Check sheet for the modelled part. Datum: model origin and axes. Units: mm. A direction names the side the tool comes from. Round coordinates to 2 decimals unless told otherwise and drop trailing zeros. Write each loop counter-clockwise with the first axis right and the second up, starting at its lowest first coordinate (ties: lowest second). Pieces come first, ordered by that corner, then holes. Notation, with made-up numbers: (2.25, 34.25) -> (60.25, 34.25) arc R19 cw to (60.25, 63.25) -> close; hole circle Ø6 at (10, -3). An arc over 180 degrees is marked (long way). Write item = value, one per line.
from build123d import *

# Parameters (mm, degrees)
CHAMFER1_SIZE      = 0.993775
CHAMFER2_SIZE      = 0.46434375
CHAMFER3_SIZE      = 0.2032
CUT_EXTRUDE2_DEPTH = 3.175


with BuildPart() as part:
    # Sketch1 → Revolve1 (revolve)
    with BuildSketch(Plane(origin=(0, 0, 0), x_dir=(0, 0, -1), z_dir=(1, 0, 0))):
        Polygon((0, 7.14375), (6.35, 7.14375), (6.35, 4.7625), (69.85, 4.7625), (69.85, 3.9751), (82.55, 3.9751), (82.55, 0), (0, 0), align=None)
    revolve(axis=Axis((0, 0, -82.55), (0, 0, 1)))

    # Sketch5 → Cut-Revolve1 (revolve, cut)
    with BuildSketch(Plane(origin=(0, 0, 0), x_dir=(0, 0, -1), z_dir=(1, 0, 0))):
        with BuildLine():
            Line((69.85, 4.7625), (74.422, 4.7625))
            Line((74.422, 4.7625), (72.6694, 3.0099))
            Line((72.6694, 3.0099), (70.8152, 3.0099))
            ThreePointArc((70.8152, 3.0099), (70.132700535, 3.292600535), (69.85, 3.9751))
            Line((69.85, 3.9751), (69.85, 4.7625))
        make_face()
    revolve(axis=Axis((0, 0, -82.55), (0, 0, 1)), mode=Mode.SUBTRACT)

    # Chamfer1
    chamfer1_edges = [part.edges().sort_by_distance(p)[0] for p in [
        (0, -3.9751, -82.55),
    ]]
    chamfer(chamfer1_edges, length=CHAMFER1_SIZE)

    # Chamfer2
    chamfer2_edges = [part.edges().sort_by_distance(p)[0] for p in [
        (0, -7.14375, 0),
    ]]
    chamfer(chamfer2_edges, length=CHAMFER2_SIZE)

    # Chamfer3
    chamfer3_edges = [part.edges().sort_by_distance(p)[0] for p in [
        (0, -4.7625, -69.85),
    ]]
    chamfer(chamfer3_edges, length=CHAMFER3_SIZE)

    # Sketch8 → Cut-Extrude2 (cut)
    with BuildSketch(Plane.XY):
        Polygon((2.38125, 1.374815329), (0, 2.749630657), (-2.38125, 1.374815329), (-2.38125, -1.374815329), (0, -2.749630657), (2.38125, -1.374815329), align=None)
    extrude(amount=-CUT_EXTRUDE2_DEPTH, mode=Mode.SUBTRACT)

    # Cut-Extrude4 cone 1 section (through the dimple's axis) → Cut-Extrude4 (revolve, cut)
    with BuildSketch(Plane(origin=(0, 0, 0), x_dir=(0, -1, 0), z_dir=(1, 0, 0))):
        Polygon((0, 0), (2.749630657, 0), (0, 2.749630657), align=None)
    revolve(axis=Axis((0, 0, 0), (0, 0, -1)), mode=Mode.SUBTRACT)

    # Sketch12 → Revolve2 (revolve)
    with BuildSketch(Plane(origin=(0, 0, 0), x_dir=(0, 0, -1), z_dir=(1, 0, 0))):
        with BuildLine():
            Line((69.85, 4.5593), (69.6468, 4.7625))
            Line((69.6468, 4.7625), (6.35, 4.7625))
            Line((6.35, 4.7625), (6.35, 0))
            Line((6.35, 0), (69.85, 0))
            Line((69.85, 0), (72.6694, 0))
            Line((72.6694, 0), (72.6694, 3.0099))
            Line((72.6694, 3.0099), (70.8152, 3.0099))
            ThreePointArc((70.8152, 3.0099), (70.132700535, 3.292600535), (69.85, 3.9751))
            Line((69.85, 3.9751), (69.85, 4.5593))
        make_face()
    revolve(axis=Axis((0, 0, -6.35), (0, 0, -1)))


solid = part.part
(1) Sectioned sample at B-B on z = -33.5. Enter the section's corners in (x, y) (1 decimal).
Worked answers:
outline = circle Ø9.5 at (0, 0)
(2) Access from +Z, -Z, +X, -X, +Y, -Y to the whole of each face (thin tool, end or side, straight path). Record for faces 1 (the flat face through (0, -3, 0)), 2 (the flat face through (1.174, -2.072, -1.565)), 3 (the cylindrical face through (3.88, -0.86, -77.65)).
Worked answers:
face_1 = +Z, +X, -X, +Y, -Y
face_2 = +Z
face_3 = -Z
(3) Release check for a two-part mould opening along Z. For faces 4 (the cylindrical face through (1.83, -2.39, -71.73)), 5 (the conical face through (-1.298, 2.21, -0.187)), 6 (the cylindrical face through (2.9, -3.78, -38.44)) record: pulls with the +Z half, pulls with the -Z half, needs draft (parallel to the pull), parting line crosses it, or undercut.
Worked answers:
face_4 = undercut
face_5 = pulls with the +Z half
face_6 = needs draft
(4) Go/stop test with flat-tipped pins: P1, Ø8, axis at y = 2, z = -18.5, coming from the +X side; P2, Ø6, axis at x = 2.5, z = -42, coming from the -Y side; P3, Ø6, axis at x = -5, z = -18.5, coming from the +Y side. Record where each tip stops, or that it passes through.
Worked answers:
P1 = 4.76
P2 = -4.76
P3 = 4.32
(5) Sectioned sample at C-C on z = -75. Enter the section's corners in (x, y).
Worked answers:
outline = circle Ø7.95 at (0, 0)
(6) Material ranges on L1, parallel to Z at x = -3.75, y = -4.75; L2, parallel to Y at x = 0.5, z = -72; L3, parallel to Z at x = -3.5, y = 0.5, recorded low to high. Write a range as [from, to].
Worked answers:
L1 = [-6.35, 0]
L2 = [-2.97, 2.97]
L3 = [-82, -73.2], [-69.96, 0]
